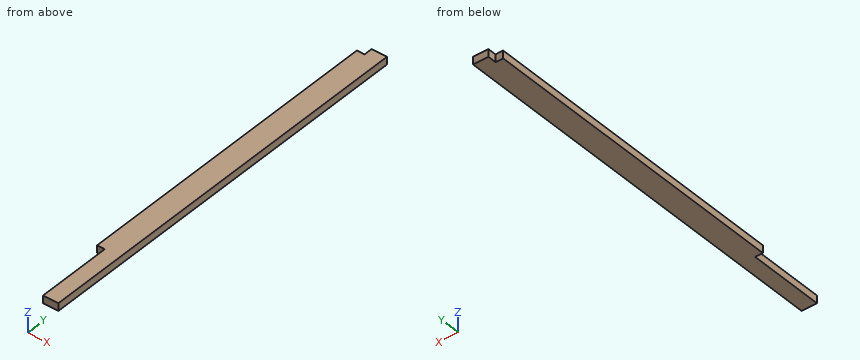
```python
from build123d import *

# Parameters (mm, degrees)
BOSS_EXTRUDE1_DEPTH = 5.4102
SKETCH2_W           = 10.8204
SKETCH2_H           = 40.64
BOSS_EXTRUDE2_DEPTH = 5.4102


with BuildPart() as part:
    # Sketch1 → Boss-Extrude1 (new body)
    with BuildSketch(Plane.XY):
        Polygon((-2.7051, -108.6104), (-2.7051, -121.158), (8.1153, -121.158), (8.1153, 121.158), (-2.7051, 121.158), (-2.7051, 114.9604), (-8.1153, 114.9604), (-8.1153, -108.6104), align=None)
    extrude(amount=BOSS_EXTRUDE1_DEPTH)

    # Sketch2 → Boss-Extrude2 (add)
    with BuildSketch(Plane.XY.offset(5.4102)):
        with Locations((2.7051, -141.478)):
            Rectangle(SKETCH2_W, SKETCH2_H)
    extrude(amount=-BOSS_EXTRUDE2_DEPTH)


solid = part.part
```
Source: CAD feature listing. Evaluate the final solid. Frame: model axes, mm. Round coordinates to 2 decimals unless told otherwise and drop trailing zeros. Loops run counter-clockwise (first coordinate to the right, second up) from the corner with the lowest first, then second, coordinate; pieces in that order, holes last.
1. Contact query for flat-ended pins moving along their axis: pin 1 (2 mm diameter, centred on x = -5, z = 1.5, fed in from -Y); pin 2 (1.6 mm diameter, centred on y = 117, z = 3.5, fed in from -X); pin 3 (1.6 mm diameter, centred on x = -6, z = 3.5, fed in from +Y). Output: stop coordinate, or through.
2. Ray query, L1, parallel to Y at x = -6.25, z = 3.65; L2, parallel to X at y = -140, z = 3.65. Return the intervals inside material, ascending.
3. Section query A-A on z = 2.25. Output: boundary loops of the cut face in (x, y), and give its area (3 significant figures).
4. Section query B-B on y = -141.5. Output: boundary loops of the cut face in (x, z).
Answers below:
1. pin 1: stops at y = -108.61
1. pin 2: stops at x = -2.71
1. pin 3: stops at y = 114.96
2. L1: y = -108.61 to 114.96
2. L2: x = -2.71 to 8.12
3. outline: (-8.12, -108.61) - (-2.71, -108.61) - (-2.71, -161.8) - (8.12, -161.8) - (8.12, 121.16) - (-2.71, 121.16) - (-2.71, 114.96) - (-8.12, 114.96) - close
3. area: 4,270 mm2
4. outline: (-2.71, 0) - (8.12, 0) - (8.12, 5.41) - (-2.71, 5.41) - close
